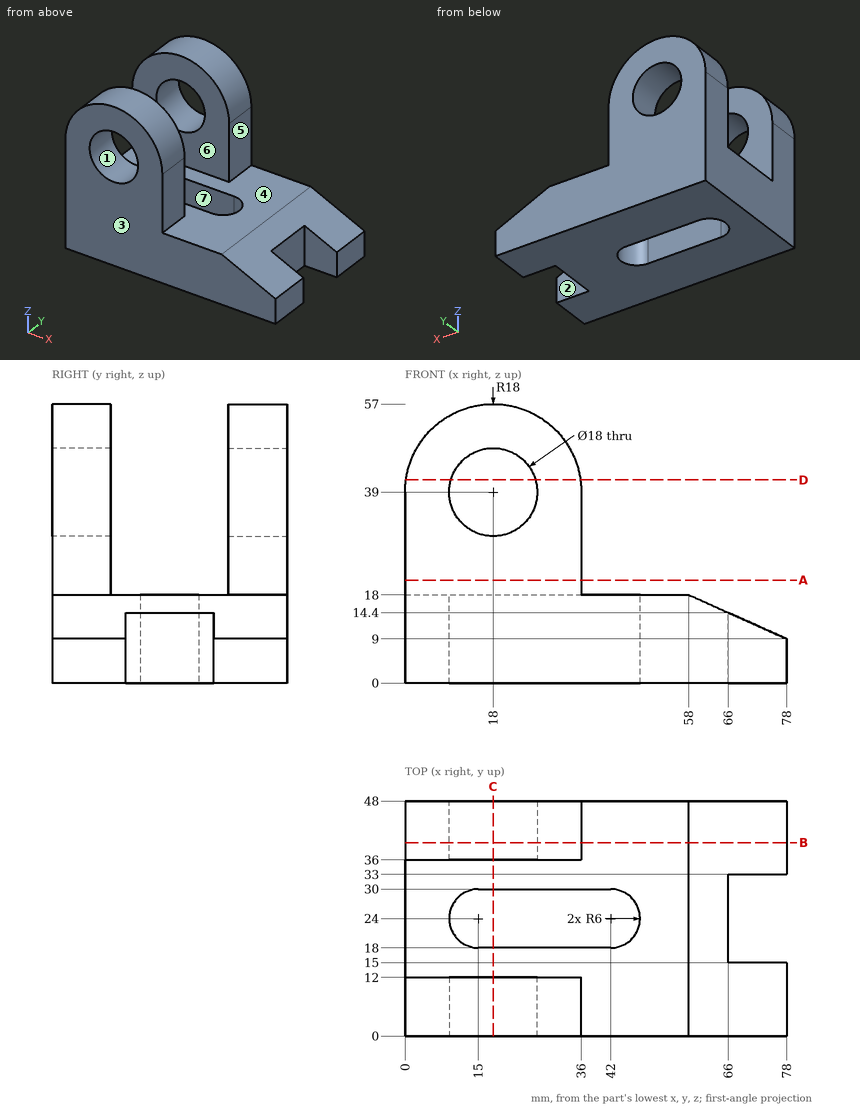
Geometry: see drawing. Coordinates: mm, zero at the bounding-box minimum. A direction names the side the tool comes from. Give positions to 0.01 mm unless a question says otherwise; leave off trailing zeros. Loops run counter-clockwise (first coordinate to the right, second up) from the corner with the lowest first, then second, coordinate; pieces in that order, holes last. Notation, with made-up numbers: M 77,65 L 98,65 A23 cw 98,87 Z; hole C -14,31.25 d7. An arc over 180 degrees is marked long. Answer as CSV lines item,"result". Start each with the question number.
1. Section A-A on z = 21. Return loops of the section in (x, y).
2. Section D-D on z = 41.5. Return loops of the section in (x, y).
3. Section C-C on x = 18. Return loops of the section in (y, z).
4. Reachability of the marked faces 5, 6 and 7 from +Z, -Z, +X, -X, +Y, -Y: full face, straight path, thin tool, end or side. Return the list, or none.
5. Section B-B on y = 39.5. Return loops of the section in (x, z), plus the area to 3 significant figures.
6. Pull-direction query (Y, two-part tool) for the marked faces 1, 2, 3 and 4; classes: released by +Y, released by -Y, zero draft, split by the parting line, or undercut.
7. Pin query (flat end, axial travel): P1, Ø1.5, axis at y = 11.5, z = 28.5, coming from the +X side; P2, Ø11, axis at x = 18, z = 39, coming from the +Y side; P3, Ø6, axis at x = 48, y = 41, coming from the +Z side; P4, Ø5, axis at y = 8.5, z = 16, coming from the +X side. Return the tip coordinate at first contact, or that it passes through.
8. Line query: L1, parallel to Y at x = 14, z = 22.5; L2, parallel to Z at x = 18, y = 40; L3, parallel to X at y = 44, z = 39. Output: solid intervals per line, ascending.
Computed values:
1,outline,"M 0,0 L 36,0 L 36,12 L 0,12 Z; M 0,36 L 36,36 L 36,48 L 0,48 Z"
2,outline,"M 0.17,0 L 9.35,0 L 9.35,12 L 0.17,12 Z; M 0.17,36 L 9.35,36 L 9.35,48 L 0.17,48 Z; M 26.65,0 L 35.83,0 L 35.83,12 L 26.65,12 Z; M 26.65,36 L 35.83,36 L 35.83,48 L 26.65,48 Z"
3,outline,"M 0,0 L 18,0 L 18,18 L 12,18 L 12,30 L 0,30 Z; M 0,48 L 12,48 L 12,57 L 0,57 Z; M 30,0 L 48,0 L 48,30 L 36,30 L 36,18 L 30,18 Z; M 36,48 L 48,48 L 48,57 L 36,57 Z"
4,face 5,"+Z, +X, +Y, -Y"
4,face 6,"+Z, +X, -X"
4,face 7,"+Z, -Z"
5,outline,"M 0,0 L 78,0 L 78,9 L 58,18 L 36,18 L 36,39 A18 ccw 0,39 Z; hole C 18,39 d18"
5,area,"2,320 mm²"
6,face 1,"zero draft"
6,face 2,"undercut"
6,face 3,"released by -Y"
6,face 4,"undercut"
7,P1,"stops at x = 36"
7,P2,"passes through"
7,P3,"stops at z = 18"
7,P4,"stops at x = 68"
8,L1,"y = 0 to 12, 36 to 48"
8,L2,"z = 0 to 30, 48 to 57"
8,L3,"x = 0 to 9, 27 to 36"
